Here's how the part is built. I have some questions about the finished solid (model axes, mm). A direction names the side the tool comes from. Give positions to 0.01 mm unless a question says otherwise; leave off trailing zeros. Write each loop counter-clockwise with the first axis right and the second up, starting at its lowest first coordinate (ties: lowest second). Pieces come first, ordered by that corner, then holes. Notation, with made-up numbers: (-18.75, -16) -> (39.25, -16) arc R23 ccw to (39.25, 18) -> close; hole circle Ø5 at (-8, 20.25). An arc over 180 degrees is marked (long way). Return JSON: item names as keys, results as strings.
from build123d import *

# Parameters (mm, degrees)
SKETCH1_W           = 11.1125
SKETCH1_H           = 3.81
BOSS_EXTRUDE1_DEPTH = 2.54
CHAMFER1_SIZE       = 2.54
CHAMFER1_SIZE_2     = 1.778527147
CHAMFER2_SIZE       = 0.680590949
CHAMFER2_SIZE_2     = 2.54
SKETCH2_W           = 6.35
SKETCH2_H           = 1.5875
BOSS_EXTRUDE2_DEPTH = 3.175


with BuildPart() as part:
    # Sketch1 → Boss-Extrude1 (new body)
    with BuildSketch(Plane.XY):
        with Locations((77.94625, 65.532)):
            Rectangle(SKETCH1_W, SKETCH1_H)
    extrude(amount=BOSS_EXTRUDE1_DEPTH)

    # Chamfer1
    # the kernel refuses this chamfer: 2.54, 1.778527147 mm, written as the material it takes off along each edge
    with BuildSketch(Plane(origin=(72.39, 73.996682665, 2.54), x_dir=(-0.02220967419845826, 0, -0.9997533347641299), z_dir=(0, -1, 0))) as chamfer1_piece_1:
        Polygon((CHAMFER1_SIZE * 0.999753334764, CHAMFER1_SIZE * 0.0222096741985), (-CHAMFER1_SIZE_2 * 0.0222096741991, CHAMFER1_SIZE_2 * 0.999753334794), (0, 0), align=None)
    extrude(amount=16.92936533, mode=Mode.SUBTRACT)

    # Chamfer2
    # the kernel refuses this chamfer: 2.54, 0.680590949 mm, written as the material it takes off along each edge
    with BuildSketch(Plane(origin=(67.572854359, 63.627, 2.54), x_dir=(0, 0.9905000388259545, 0.13751244702128823), z_dir=(1, 0, 0))) as chamfer2_piece_1:
        Polygon((CHAMFER2_SIZE * 0.990500038499, -CHAMFER2_SIZE * 0.137512446976), (-CHAMFER2_SIZE_2 * 0.137512447021, -CHAMFER2_SIZE_2 * 0.990500038826), (0, 0), align=None)
    extrude(amount=22.52531843, mode=Mode.SUBTRACT)
    with BuildSketch(Plane(origin=(83.5025, 57.031327212, 2.54), x_dir=(-0.9905000388259543, 0, 0.13751244702128956), z_dir=(0, 1, 0))) as chamfer2_piece_2:
        Polygon((CHAMFER2_SIZE * 0.990500038499, -CHAMFER2_SIZE * 0.137512446976), (-CHAMFER2_SIZE_2 * 0.137512447021, -CHAMFER2_SIZE_2 * 0.990500038826), (0, 0), align=None)
    extrude(amount=17.001345577, mode=Mode.SUBTRACT)
    with BuildSketch(Plane(origin=(90.098172788, 67.437, 2.54), x_dir=(0, 0.009967146577158238, -0.9999503267608394), z_dir=(-1, 0, 0))) as chamfer2_piece_3:
        Polygon((CHAMFER2_SIZE_2 * 0.999950326761, CHAMFER2_SIZE_2 * 0.00996714657716), (-CHAMFER2_SIZE * 0.00996714657386, CHAMFER2_SIZE * 0.99995032643), (0, 0), align=None)
    extrude(amount=22.52531843, mode=Mode.SUBTRACT)

    # Sketch2 → Boss-Extrude2 (add)
    with BuildSketch(Plane(origin=(0, 0, 0), x_dir=(-1, 0, 0), z_dir=(0, 0, -1))):
        with Locations((-77.94625, 65.532)):
            Rectangle(SKETCH2_W, SKETCH2_H)
    extrude(amount=BOSS_EXTRUDE2_DEPTH)


solid = part.part
1. For pin 1 Ø0.5 at (y, z) = (66, -1) entering from -X; pin 2 Ø2.5 at (x, z) = (77.5, -2) entering from +Y; pin 3 Ø1 at (x, z) = (78, -1) entering from -Y, each with a flat end and sliding along its axis, tell me the tip position at first contact or that it passes through.
Taken from the geometry:
{"pin 1": "stops at x = 74.77", "pin 2": "stops at y = 66.33", "pin 3": "stops at y = 64.74"}
2. If I drill on line 1 (Z direction, x = 82, y = 66.7); line 2 (Y direction, x = 75, z = -2.5); line 3 (X direction, y = 66.15, z = -0.75), over which ranges is the centre line in solid material (lowest first)? Write a range as [from, to].
Taken from the geometry:
{"line 1": "z = [0, 2.54]", "line 2": "y = [64.74, 66.33]", "line 3": "x = [74.77, 81.12]"}
3. Suppose I cut it at B-B, the plane x = 77.25. List the corners of the cut face in (y, z) for me (3 decimals), and give its area (3 significant figures).
Taken from the geometry:
{"outline": "(63.627, 0) -> (64.738, 0) -> (64.738, -3.175) -> (66.326, -3.175) -> (66.326, 0) -> (67.437, 0) -> (66.756, 2.54) -> (64.308, 2.54) -> close", "area": "13.0 mm²"}
4. Which directions (+Z, -Z, +X, -X, +Y, -Y) give clear straight access to the entire face, cutting with the end or side of a thin tool? Please do faces 1 (the face through (74.771, 66, -2)), 2 (the face through (78, 66.326, -2)), 3 (the face through (81.121, 66, -2)), 4 (the face through (78, 64.738, -2)).
Taken from the geometry:
{"face 1": "-Z, -X, +Y, -Y", "face 2": "-Z, +X, -X, +Y", "face 3": "-Z, +X, +Y, -Y", "face 4": "-Z, +X, -X, -Y"}
5. Suppose I cut it at D-D, the plane x = 74.5. List the corners of the cut face in (y, z) for me, and give its area (3 significant figures).
Taken from the geometry:
{"outline": "(63.63, 0) -> (67.44, 0) -> (66.76, 2.54) -> (64.31, 2.54) -> close", "area": "7.95 mm²"}
6. Suppose I cut it at A-A, the plane y = 65.8. List the corners of the cut face in (x, z) for me (1 decimal).
Taken from the geometry:
{"outline": "(72.4, 0) -> (74.8, 0) -> (74.8, -3.2) -> (81.1, -3.2) -> (81.1, 0) -> (83.5, 0) -> (82.8, 2.5) -> (74.2, 2.5) -> close"}
7. Suppose I cut it at C-C, the plane z = -2.7. List the corners of the cut face in (x, y) for me, and give its area (3 significant figures).
Taken from the geometry:
{"outline": "(74.77, 64.74) -> (81.12, 64.74) -> (81.12, 66.33) -> (74.77, 66.33) -> close", "area": "10.1 mm²"}
